The listing builds one solid part. Answer for the finished solid, in the listing's coordinates (mm). A direction names the side the tool comes from. Give positions to 0.01 mm unless a question says otherwise; leave off trailing zeros. Order: outer loops, then holes, each group sorted by start corner. A loop starts at its lowest first (then second) coordinate and runs counter-clockwise, first axis right, second up. Notation, with made-up numbers: (67.25, 13.25) - (90.25, 13.25) arc R33 ccw to (90.25, 51.25) - close; hole circle Ø9 at (60.5, -16). An arc over 180 degrees is marked (long way). Answer as a JSON object with one key per item and string values. Group by question number.
Q1. A cutting plane is placed at A-A, the plane y = -6.3. Give the vertices of the cut face in (x, z).
Q2. A cutting plane is placed at C-C, the plane z = 7. Count the separate pieces of the cut face and the enclosed holes in it, and give its area (3 significant figures).
Q3. For faces 1 (the face through (0, -11.15, 5)), 2 (the face through (26, 0, 9.775)), 3 (the face through (0, 0, 4.4)), 4 (the face through (-21, 11.2, 9.9)), determine the directions among +Z, -Z, +X, -X, +Y, -Y from which every point of the face is accessible in a straight line to the end or side of a thin tool.
Q4. Given pin 1 (0.8 mm diameter, centred on x = -23.5, y = 12, fed in from +Z); pin 2 (1.2 mm diameter, centred on x = -7, y = -0.5, fed in from +Z); pin 3 (0.9 mm diameter, centred on y = 0, z = 6, fed in from +X), each flat-ended and moving along its own axis, determine where each tip first touches the part or whether it passes through.
Q5. A cutting plane is placed at B-B, the plane y = 2. Give the vertices of the cut face in (x, z).
Q6. The mould has two halves that part along Z. Classify faces 5 (the face through (-26.5, 0, 6)), 6 (the face through (24, -12, 8.3)), 7 (the face through (24.5, 0, 6)), 8 (the face through (26.01, 8.87, 9.8)): released by +Z, released by -Z, zero draft, split by the parting line, or undercut.
Q7. Consider line 1 (Y direction, x = 23.5, z = 3.25); line 2 (Y direction, x = 26, z = 7); line 3 (Y direction, x = -24.9, z = 7). Determine where each line is inside the solid, lowest interval first.
from build123d import *

# Parameters (mm, degrees)
SKICA1_W                 = 53
SKICA1_H                 = 24.4
P_IDAT_VYSUNUT_M1_DEPTH  = 2.5
SKICA2_W                 = 49
SKICA2_H                 = 1.05
P_IDAT_VYSUNUT_M2_DEPTH  = 9.3
SKICA3_W                 = 16.2
SKICA3_H                 = 1.05
SKICA3_W_2               = 1.9
ODEBRAT_VYSUNUT_M1_DEPTH = 3.5
SKICA7_W                 = 14.5
SKICA7_H                 = 3.5
P_IDAT_VYSUNUT_M3_DEPTH  = 2.6
SKICA6_W                 = 14.5
SKICA6_H                 = 3.5
P_IDAT_VYSUNUT_M4_DEPTH  = 2.6
SKICA8_W                 = 14.5
SKICA8_H                 = 3.5
P_IDAT_VYSUNUT_M5_DEPTH  = 2.6
ZAOBLIT3_R               = 3.5
ODEBRAT_START            = -45.2
ODEBRAT_VYSUNUT_M2_DEPTH = 45.2
ODEBRAT_VYSUNUT_M3_DEPTH = 45.2
ZKOSEN_3_SIZE            = 3.5
SKICA14_W                = 2
SKICA14_H                = 24.4
P_IDAT_VYSUNUT_M6_DEPTH  = 10.05
ZAOBLIT4_R               = 4.25
SKICA17_W                = 7
SKICA17_H                = 1.9
ODEBRAT_VYSUNUT_M4_DEPTH = 2.05
SKICA18_R                = 3.8
ODEBRAT_VYSUNUT_M5_DEPTH = 1
SKICA20_R                = 1.25
ODEBRAT_VYSUNUT_M6_DEPTH = 1
ODEBRAT_START_2          = -1
SKICA21_R                = 3.8
ODEBRAT_VYSUNUT_M7_DEPTH = 1
SKICA22_R                = 1.25
ODEBRAT_VYSUNUT_M8_DEPTH = 1
SKICA23_W                = 49
SKICA23_H                = 1.1
P_IDAT_VYSUNUT_M7_DEPTH  = 9.7
SKICA24_W                = 26
SKICA24_H                = 1.1
ODEBRAT_VYSUNUT_M9_DEPTH = 7.8


with BuildPart() as part:
    # Skica1 → Přidat vysunutím1 (new body)
    with BuildSketch(Plane.XY):
        Rectangle(SKICA1_W, SKICA1_H)
    extrude(amount=P_IDAT_VYSUNUT_M1_DEPTH)

    # Skica2 → Přidat vysunutím2 (add)
    with BuildSketch(Plane.XY.offset(2.5)):
        with Locations((0, 11.675)):
            Rectangle(SKICA2_W, SKICA2_H)
        with Locations((0, -11.675)):
            Rectangle(SKICA2_W, SKICA2_H)
    extrude(amount=P_IDAT_VYSUNUT_M2_DEPTH)

    # Skica3 → Odebrat vysunutím1 (cut)
    with BuildSketch(Plane.XY.offset(11.8)):
        with Locations((0, -11.675)):
            Rectangle(SKICA3_W, SKICA3_H)
        with Locations((0, 11.675)):
            Rectangle(SKICA3_W, SKICA3_H)
        with Locations((-23.55, 11.675)):
            Rectangle(SKICA3_W_2, SKICA3_H)
        with Locations((-23.55, -11.675)):
            Rectangle(SKICA3_W_2, SKICA3_H)
        with Locations((23.55, 11.675)):
            Rectangle(SKICA3_W_2, SKICA3_H)
        with Locations((23.55, -11.675)):
            Rectangle(SKICA3_W_2, SKICA3_H)
    extrude(amount=-ODEBRAT_VYSUNUT_M1_DEPTH, mode=Mode.SUBTRACT)

    # Skica7 → Přidat vysunutím3 (add)
    with BuildSketch(Plane(origin=(0, 11.15, 0), x_dir=(-1, 0, 0), z_dir=(0, -1, 0))):
        with Locations((15.35, -10.05)):
            Rectangle(SKICA7_W, SKICA7_H)
        with Locations((-15.35, -10.05)):
            Rectangle(SKICA7_W, SKICA7_H)
    extrude(amount=P_IDAT_VYSUNUT_M3_DEPTH)

    # Skica6 → Přidat vysunutím4 (add)
    with BuildSketch(Plane(origin=(0, -11.15, 0), x_dir=(1, 0, 0), z_dir=(0, 1, 0))):
        with Locations((-15.35, -10.05)):
            Rectangle(SKICA6_W, SKICA6_H)
    extrude(amount=P_IDAT_VYSUNUT_M4_DEPTH)

    # Skica8 → Přidat vysunutím5 (add)
    with BuildSketch(Plane(origin=(0, -11.15, 0), x_dir=(1, 0, 0), z_dir=(0, 1, 0))):
        with Locations((15.35, -10.05)):
            Rectangle(SKICA8_W, SKICA8_H)
    extrude(amount=P_IDAT_VYSUNUT_M5_DEPTH)

    # Zaoblit3
    zaoblit3_edges = [part.edges().sort_by_distance(p)[0] for p in [
        (15.35, 12.2, 11.8),
        (-15.35, 12.2, 11.8),
        (-15.35, -12.2, 11.8),
        (15.35, -12.2, 11.8),
    ]]
    fillet(zaoblit3_edges, radius=ZAOBLIT3_R)

    # Skica11 → Odebrat vysunutím2 (cut)
    with BuildSketch(Plane(origin=(22.6, 0, 0), x_dir=(0, 0, -1), z_dir=(1, 0, 0)).offset(ODEBRAT_START)):
        with BuildLine():
            Line((-11.8, -8.55), (-8.3, -8.55))
            Line((-8.3, -8.55), (-8.3, -11.15))
            add(Edge.make_bspline(
                [(-8.3, -11.15), (-11.489612279, -10.573938185), (-11.8, -8.55)],
                knots=[0, 0, 0, 0.822635588, 0.822635588, 0.822635588], degree=2))
        make_face()
    extrude(amount=ODEBRAT_VYSUNUT_M2_DEPTH, mode=Mode.SUBTRACT)

    # Skica13 → Odebrat vysunutím3 (cut)
    with BuildSketch(Plane(origin=(22.6, 0, 0), x_dir=(0, 0, -1), z_dir=(1, 0, 0)).offset(ODEBRAT_START)):
        with BuildLine():
            Line((-11.8, 8.55), (-8.3, 8.55))
            Line((-8.3, 8.55), (-8.3, 11.15))
            add(Edge.make_bspline(
                [(-8.3, 11.15), (-11.594475323, 10.62667069), (-11.8, 8.55)],
                knots=[0, 0, 0, 0.882557327, 0.882557327, 0.882557327], degree=2))
        make_face()
    extrude(amount=ODEBRAT_VYSUNUT_M3_DEPTH, mode=Mode.SUBTRACT)

    # Zkosení3
    # the kernel refuses this chamfer: 3.5 mm, written as the material it takes off along each edge
    with BuildSketch(Plane(origin=(-22.6, 0.450890458, 11.8), x_dir=(-0.027495876610586112, 0, -0.9996219169112968), z_dir=(0, -1, 0)), Plane(origin=(-8.1, 0.450890458, 11.8), x_dir=(-0.9996219169112968, 0, 0.027495876610586605), z_dir=(0, -1, 0)), Plane(origin=(-22.6, -0.450890458, 11.8), x_dir=(0.9996219169112968, 3.891912830509087e-15, 0.02749587661058662), z_dir=(0, 1, 0)), Plane(origin=(-8.1, -0.450890458, 11.8), x_dir=(0.027495876610586605, 0, -0.9996219169112968), z_dir=(0, 1, 0)), Plane(origin=(8.1, -0.450890458, 11.8), x_dir=(0.9996219169112968, 0, 0.027495876610586605), z_dir=(0, 1, 0)), Plane(origin=(22.6, -0.450890458, 11.8), x_dir=(0.027495876610586112, 0, -0.9996219169112968), z_dir=(0, 1, 0)), Plane(origin=(8.1, 0.450890458, 11.8), x_dir=(-0.027495876610586605, 0, -0.9996219169112968), z_dir=(0, -1, 0)), Plane(origin=(22.6, 0.450890458, 11.8), x_dir=(-0.9996219169112968, 3.891912830509087e-15, 0.02749587661058662), z_dir=(0, -1, 0))) as zkosen_3_piece_1:
        Polygon((ZKOSEN_3_SIZE * 0.999621916911, ZKOSEN_3_SIZE * 0.0274958766106), (-ZKOSEN_3_SIZE * 0.0274958766106, ZKOSEN_3_SIZE * 0.999621916911), (0, 0), align=None)
    extrude(amount=18.151780916, mode=Mode.SUBTRACT)

    # Skica14 → Přidat vysunutím6 (add)
    with BuildSketch(Plane.XY.offset(2.5)):
        with Locations((25.5, 0)):
            Rectangle(SKICA14_W, SKICA14_H)
        with Locations((-25.5, 0)):
            Rectangle(SKICA14_W, SKICA14_H)
    extrude(amount=P_IDAT_VYSUNUT_M6_DEPTH)

    # Zaoblit4
    zaoblit4_edges = [part.edges().sort_by_distance(p)[0] for p in [
        (-25.5, 12.2, 12.55),
        (-25.5, -12.2, 12.55),
        (25.5, -12.2, 12.55),
        (25.5, 12.2, 12.55),
    ]]
    fillet(zaoblit4_edges, radius=ZAOBLIT4_R)

    # Skica17 → Odebrat vysunutím4 (cut)
    with BuildSketch(Plane(origin=(26.5, 0, 0), x_dir=(0, 0, -1), z_dir=(1, 0, 0))):
        with Locations((-6.275, 0)):
            Rectangle(SKICA17_W, SKICA17_H)
    extrude(amount=-ODEBRAT_VYSUNUT_M4_DEPTH, mode=Mode.SUBTRACT)

    # Skica18 → Odebrat vysunutím5 (cut)
    with BuildSketch(Plane(origin=(26.5, 0, 0), x_dir=(0, 0, -1), z_dir=(1, 0, 0))):
        with Locations((-7, 6.3)):
            Circle(SKICA18_R)
        with Locations((-7, -6.3)):
            Circle(SKICA18_R)
    extrude(amount=-ODEBRAT_VYSUNUT_M5_DEPTH, mode=Mode.SUBTRACT)

    # Skica20 → Odebrat vysunutím6 (cut)
    with BuildSketch(Plane(origin=(25.5, 0, 0), x_dir=(0, 0, -1), z_dir=(1, 0, 0))):
        with Locations((-7, -6.3)):
            Circle(SKICA20_R)
        with Locations((-7, 6.3)):
            Circle(SKICA20_R)
    extrude(amount=-ODEBRAT_VYSUNUT_M6_DEPTH, mode=Mode.SUBTRACT)

    # Skica21 → Odebrat vysunutím7 (cut)
    with BuildSketch(Plane.ZY.offset(26.5).offset(ODEBRAT_START_2)):
        with Locations(Location((7, 6.3, 0), (0, 0, 180))):
            Circle(SKICA21_R)
        with Locations(Location((7, -6.3, 0), (0, 0, 180))):
            Circle(SKICA21_R)
    extrude(amount=ODEBRAT_VYSUNUT_M7_DEPTH, mode=Mode.SUBTRACT)

    # Skica22 → Odebrat vysunutím8 (cut)
    with BuildSketch(Plane.ZY.offset(25.5).offset(ODEBRAT_START_2)):
        with Locations(Location((7, -6.3, 0), (0, 0, 180))):
            Circle(SKICA22_R)
        with Locations(Location((7, 6.3, 0), (0, 0, 180))):
            Circle(SKICA22_R)
    extrude(amount=ODEBRAT_VYSUNUT_M8_DEPTH, mode=Mode.SUBTRACT)

    # Skica23 → Přidat vysunutím7 (add)
    with BuildSketch(Plane.XY.offset(2.5)):
        Rectangle(SKICA23_W, SKICA23_H)
    extrude(amount=P_IDAT_VYSUNUT_M7_DEPTH)

    # Skica24 → Odebrat vysunutím9 (cut)
    with BuildSketch(Plane.XY.offset(12.2)):
        Rectangle(SKICA24_W, SKICA24_H)
    extrude(amount=-ODEBRAT_VYSUNUT_M9_DEPTH, mode=Mode.SUBTRACT)

    # Zkosení5
    # the kernel refuses this chamfer: 11.5 mm, written as the material it takes off along each edge
    with BuildSketch(Plane(origin=(-13, -0.55, 12.2), x_dir=(-0.9996219169112968, 0, 0.027495876610586382), z_dir=(0, 1, 0))) as zkosen_5_piece_1_section:
        with BuildLine():
            Line((11.829741745, 0), (-0.650292281, -11.811854626))
            Line((-0.650292281, -11.811854626), (-0.880205322, -11.805530574))
            ThreePointArc((-0.880205322, -11.805530574), (-0.392486111, -5.904075041), (-0.229913041, 0.006324052))
            Line((-0.229913041, 0.006324052), (0.006324052, 0.229913041))
            ThreePointArc((0.006324052, 0.229913041), (5.916723144, 0.067339971), (11.836065796, 0.229913041))
            Line((11.836065796, 0.229913041), (11.829741745, 0))
        make_face()
    zkosen_5_piece_1 = extrude(amount=1.1, mode=Mode.PRIVATE)
    zkosen_5_piece_1 = split(zkosen_5_piece_1, bisect_by=Plane(origin=(-24.5, 0, 9.11358538), z_dir=(1, 0, 0)), keep=Keep.TOP, mode=Mode.PRIVATE)
    zkosen_5_piece_1 = split(zkosen_5_piece_1, bisect_by=Plane(origin=(-17.151338027, 0, 4.4), z_dir=(0, 0, 1)), keep=Keep.TOP, mode=Mode.PRIVATE)
    add(zkosen_5_piece_1, mode=Mode.SUBTRACT)

    # Zkosení6
    # the kernel refuses this chamfer: 11.5 mm, written as the material it takes off along each edge
    with BuildSketch(Plane(origin=(13, 0.55, 12.2), x_dir=(-0.02749587661058638, 0, -0.9996219169112968), z_dir=(0, -1, 0))) as zkosen_6_piece_1_section:
        with BuildLine():
            Line((11.829741745, 0), (-0.650292281, 11.811854626))
            Line((-0.650292281, 11.811854626), (-0.880205322, 11.805530574))
            ThreePointArc((-0.880205322, 11.805530574), (-0.392486111, 5.904075041), (-0.229913041, -0.006324052))
            Line((-0.229913041, -0.006324052), (0.006324052, -0.229913041))
            ThreePointArc((0.006324052, -0.229913041), (5.916723144, -0.067339971), (11.836065796, -0.229913041))
            Line((11.836065796, -0.229913041), (11.829741745, 0))
        make_face()
    zkosen_6_piece_1 = extrude(amount=1.1, mode=Mode.PRIVATE)
    zkosen_6_piece_1 = split(zkosen_6_piece_1, bisect_by=Plane(origin=(24.5, 0, 9.11358538), z_dir=(-1, 0, 0)), keep=Keep.TOP, mode=Mode.PRIVATE)
    zkosen_6_piece_1 = split(zkosen_6_piece_1, bisect_by=Plane(origin=(17.151338027, 0, 4.4), z_dir=(0, 0, 1)), keep=Keep.TOP, mode=Mode.PRIVATE)
    add(zkosen_6_piece_1, mode=Mode.SUBTRACT)


solid = part.part
Reply:
{
 "1": {"outline": "(-26.5, 0) - (26.5, 0) - (26.5, 3.2) - (25.5, 3.2) - (25.5, 5.75) - (24.5, 5.75) - (24.5, 2.5) - (-24.5, 2.5) - (-24.5, 5.75) - (-25.5, 5.75) - (-25.5, 3.2) - (-26.5, 3.2) - close; (-26.5, 10.8) - (-25.5, 10.8) - (-25.5, 8.25) - (-24.5, 8.25) - (-24.5, 12.55) - (-26.5, 12.55) - close; (24.5, 8.25) - (25.5, 8.25) - (25.5, 10.8) - (26.5, 10.8) - (26.5, 12.55) - (24.5, 12.55) - close"},
 "2": {"separate pieces": "6", "enclosed holes": "0", "area": "168 mm^2"},
 "3": {"face 1": "none", "face 2": "+X", "face 3": "+Z", "face 4": "+Z, +Y"},
 "4": {"pin 1": "stops at z = 8.3", "pin 2": "stops at z = 4.4", "pin 3": "stops at x = 24.5"},
 "5": {"outline": "(-26.5, 0) - (26.5, 0) - (26.5, 12.55) - (24.5, 12.55) - (24.5, 2.5) - (-24.5, 2.5) - (-24.5, 12.55) - (-26.5, 12.55) - close"},
 "6": {"face 5": "zero draft", "face 6": "released by +Z", "face 7": "undercut", "face 8": "undercut"},
 "7": {"line 1": "y = -12.2 to -11.15, -0.55 to 0.55, 11.15 to 12.2", "line 2": "y = -12.2 to -10.1, -2.5 to -0.95, 0.95 to 2.5, 10.1 to 12.2", "line 3": "y = -12.2 to -7.55, -5.05 to 5.05, 7.55 to 12.2"}
}
